Here's how the part is built. I have some questions about the finished solid (model axes, mm). Give positions to 0.01 mm unless a question says otherwise; leave off trailing zeros. Order: outer loops, then holes, each group sorted by start corner. A loop starts at its lowest first (then second) coordinate and runs counter-clockwise, first axis right, second up.
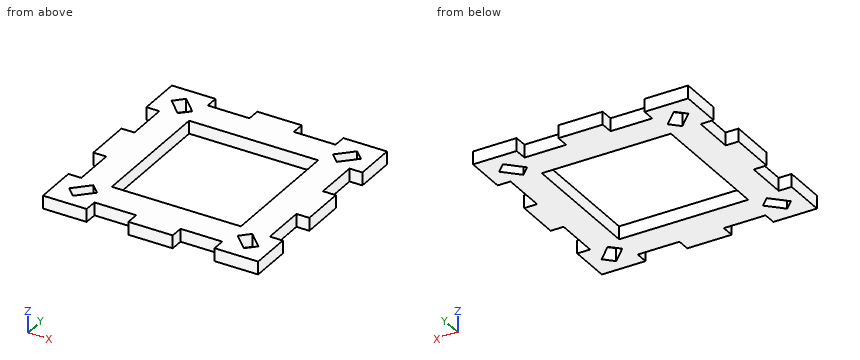
from build123d import *

# Parameters (mm, degrees)
SALIENTE_EXTRUIR1_DEPTH = 3
CROQUIS2_W              = 30
CROQUIS2_H              = 30
CORTAR_EXTRUIR2_DEPTH   = 3
CORTAR_EXTRUIR3_DEPTH   = 3


with BuildPart() as part:
    # Croquis1 → Saliente-Extruir1 (new body)
    with BuildSketch(Plane.XY):
        Polygon((-25, -25), (-14.85, -25), (-14.85, -22), (-5.15, -22), (-5.15, -25), (5.15, -25), (5.15, -22), (14.85, -22), (14.85, -25), (25, -25), (25, -15.45), (22, -15.45), (22, -5.15), (25, -5.15), (25, 5.15), (22, 5.15), (22, 15.45), (25, 15.45), (25, 25), (14.85, 25), (14.85, 22), (5.15, 22), (5.15, 25), (-5.15, 25), (-5.15, 22), (-14.85, 22), (-14.85, 25), (-25, 25), (-25, 15.15), (-22, 15.15), (-22, 5.45), (-25, 5.45), (-25, -5.45), (-22, -5.45), (-22, -15.15), (-25, -15.15), align=None)
    extrude(amount=SALIENTE_EXTRUIR1_DEPTH)

    # Croquis2 → Cortar-Extruir2 (cut)
    with BuildSketch(Plane.XY.offset(3)):
        Rectangle(CROQUIS2_W, CROQUIS2_H)
    extrude(amount=-CORTAR_EXTRUIR2_DEPTH, mode=Mode.SUBTRACT)

    # Croquis3 → Cortar-Extruir3 (cut)
    with BuildSketch(Plane.XY.offset(3)):
        Polygon((-19.878679656, -22), (-16.343145751, -18.464466094), (-18.464466094, -16.343145751), (-22, -19.878679656), align=None)
        Polygon((16.343145751, -18.464466094), (18.464466094, -16.343145751), (22, -19.878679656), (19.878679656, -22), align=None)
        Polygon((22, 19.878679656), (18.464466094, 16.343145751), (16.343145751, 18.464466094), (19.878679656, 22), align=None)
        Polygon((-22, 19.878679656), (-18.464466094, 16.343145751), (-16.343145751, 18.464466094), (-19.878679656, 22), align=None)
    extrude(amount=-CORTAR_EXTRUIR3_DEPTH, mode=Mode.SUBTRACT)


solid = part.part
Q1. I'm going to push flat-ended pins straight in: P1, Ø1.5, axis at y = 9.5, z = 1, coming from the -X side; P2, Ø0.9, axis at x = -12, z = 2, coming from the +Y side. Where does each tip first touch, or does it pass through?
Filled sheet:
P1: stops at x = -22
P2: stops at y = 22
Q2. If we section it at A-A on y = 13: List the corners of the cut face in (x, z) for me, plus the area to 3 significant figures.
Filled sheet:
outline: (-22, 0) - (-15, 0) - (-15, 3) - (-22, 3) - close; (15, 0) - (22, 0) - (22, 3) - (15, 3) - close
area: 42.0 mm2
Q3. I need wall thicknesses on L1, parallel to X at y = 13.5, z = 1.75; L2, parallel to X at y = 2, z = 2.7. Which ranges of each line are inside material? Lowest first, please.
Filled sheet:
L1: x = -22 to -15, 15 to 22
L2: x = -25 to -15, 15 to 25
Q4. If we section it at C-C on z = 0.8: Give the number of separate pieces and of enclosed holes in the cut face, plus the area to 3 significant figures.
Filled sheet:
separate pieces: 1
enclosed holes: 5
area: 1,300 mm2
Q5. If we section it at B-B on x = 3: List the corners of the cut face in (y, z) for me.
Filled sheet:
outline: (-25, 0) - (-15, 0) - (-15, 3) - (-25, 3) - close; (15, 0) - (25, 0) - (25, 3) - (15, 3) - close
